from build123d import *

# Parameters (mm, degrees)
SKETCH1_R           = 48.26
BOSS_EXTRUDE1_DEPTH = 8.89
SKETCH3_R           = 1.7145
CUT_EXTRUDE1_DEPTH  = 3.81
SKETCH4_R           = 21.0185
CUT_EXTRUDE2_DEPTH  = 8.89
CUT_EXTRUDE3_DEPTH  = 99.56230669
BOSS_EXTRUDE2_START = -1.905
SKETCH8_R           = 2
BOSS_EXTRUDE2_DEPTH = 1.905
SKETCH9_R           = 23.622
CUT_EXTRUDE4_DEPTH  = 7.0104


with BuildPart() as part:
    # Sketch1 → Boss-Extrude1 (new body)
    with BuildSketch(Plane.XY):
        with Locations((21.15, -21.15)):
            Circle(SKETCH1_R)
    extrude(amount=BOSS_EXTRUDE1_DEPTH)

    # Sketch3 → Cut-Extrude1 (cut)
    with BuildSketch(Plane.XY.offset(8.89)):
        with Locations((25.240891907, 16.090983183)):
            Circle(SKETCH3_R)
        with Locations((34.034368653, 14.02981338)):
            Circle(SKETCH3_R)
        with Locations((42.079052724, 9.924120696)):
            Circle(SKETCH3_R)
        with Locations((48.907416326, 4.012513068)):
            Circle(SKETCH3_R)
        with Locations((54.122619785, -3.361448357)):
            Circle(SKETCH3_R)
        with Locations((57.421574432, -11.769215746)):
            Circle(SKETCH3_R)
        with Locations((58.612557015, -20.722160217)):
            Circle(SKETCH3_R)
        with Locations((57.626351956, -29.699969182)):
            Circle(SKETCH3_R)
        with Locations((54.520273906, -38.180885015)):
            Circle(SKETCH3_R)
        with Locations((49.474836834, -45.672027717)):
            Circle(SKETCH3_R)
        with Locations((42.783263201, -51.738039301)):
            Circle(SKETCH3_R)
        with Locations((34.834442945, -56.026385224)):
            Circle(SKETCH3_R)
        with Locations((26.090332605, -58.287842408)):
            Circle(SKETCH3_R)
        with Locations((17.059108093, -58.390983183)):
            Circle(SKETCH3_R)
        with Locations((8.265631347, -56.32981338)):
            Circle(SKETCH3_R)
        with Locations((0.220947276, -52.224120696)):
            Circle(SKETCH3_R)
        with Locations((-6.607416326, -46.312513068)):
            Circle(SKETCH3_R)
        with Locations((-11.822619785, -38.938551643)):
            Circle(SKETCH3_R)
        with Locations((-15.121574432, -30.530784254)):
            Circle(SKETCH3_R)
        with Locations((-16.312557015, -21.577839783)):
            Circle(SKETCH3_R)
        with Locations((-15.326351956, -12.600030818)):
            Circle(SKETCH3_R)
        with Locations((-12.220273906, -4.119114985)):
            Circle(SKETCH3_R)
        with Locations((-7.174836834, 3.372027717)):
            Circle(SKETCH3_R)
        with Locations((-0.483263201, 9.438039301)):
            Circle(SKETCH3_R)
        with Locations((7.465557055, 13.726385224)):
            Circle(SKETCH3_R)
        with Locations((16.209667395, 15.987842408)):
            Circle(SKETCH3_R)
    extrude(amount=-CUT_EXTRUDE1_DEPTH, mode=Mode.SUBTRACT)

    # Sketch4 → Cut-Extrude2 (cut)
    with BuildSketch(Plane.XY.offset(8.89)):
        with Locations((21.15, -21.15)):
            Circle(SKETCH4_R)
    extrude(amount=-CUT_EXTRUDE2_DEPTH, mode=Mode.SUBTRACT)

    # Sketch5 → Cut-Extrude3 (cut, through all)
    with BuildSketch(Plane(origin=(0, 0, 0), x_dir=(-1, 0, 0), z_dir=(0, 0, -1))):
        with BuildLine():
            ThreePointArc((-24.96, 23.3), (-21.15, 19.49), (-17.34, 23.3))
            Line((-17.34, 23.3), (-17.34, 26.959370189))
            ThreePointArc((-17.34, 26.959370189), (-21.15, 27.11), (-24.96, 26.959370189))
            Line((-24.96, 26.959370189), (-24.96, 23.3))
        make_face()
        with BuildLine():
            Line((-65.6, -17.34), (-69.259370189, -17.34))
            ThreePointArc((-69.259370189, -17.34), (-69.41, -21.15), (-69.259370189, -24.96))
            Line((-69.259370189, -24.96), (-65.6, -24.96))
            ThreePointArc((-65.6, -24.96), (-61.79, -21.15), (-65.6, -17.34))
        make_face()
        with BuildLine():
            Line((-24.96, -65.6), (-24.96, -69.259370189))
            ThreePointArc((-24.96, -69.259370189), (-21.15, -69.41), (-17.34, -69.259370189))
            Line((-17.34, -69.259370189), (-17.34, -65.6))
            ThreePointArc((-17.34, -65.6), (-21.15, -61.79), (-24.96, -65.6))
        make_face()
        with BuildLine():
            ThreePointArc((27.11, -21.15), (27.072327844, -19.243511779), (26.959370189, -17.34))
            Line((26.959370189, -17.34), (23.3, -17.34))
            ThreePointArc((23.3, -17.34), (19.49, -21.15), (23.3, -24.96))
            Line((23.3, -24.96), (26.959370189, -24.96))
            ThreePointArc((26.959370189, -24.96), (27.072327844, -23.056488221), (27.11, -21.15))
        make_face()
    extrude(amount=-CUT_EXTRUDE3_DEPTH, mode=Mode.SUBTRACT)

    # Sketch8 → Boss-Extrude2 (add)
    # profile 1 of 4: a face of its own
    with BuildSketch(Plane.XY.offset(8.89).offset(BOSS_EXTRUDE2_START)):
        with BuildLine():
            ThreePointArc((-26.959370189, -17.34), (-27.11, -21.15), (-26.959370189, -24.96))
            Line((-26.959370189, -24.96), (-23.3, -24.96))
            ThreePointArc((-23.3, -24.96), (-19.49, -21.15), (-23.3, -17.34))
            Line((-23.3, -17.34), (-26.959370189, -17.34))
        make_face()
        with Locations((-23.3, -21.15)):
            Circle(SKETCH8_R, mode=Mode.SUBTRACT)
    # profile 2 of 4: a face of its own
    with BuildSketch(Plane.XY.offset(8.89).offset(BOSS_EXTRUDE2_START)):
        with BuildLine():
            ThreePointArc((24.96, 26.959370189), (21.15, 27.11), (17.34, 26.959370189))
            Line((17.34, 26.959370189), (17.34, 23.3))
            ThreePointArc((17.34, 23.3), (21.15, 19.49), (24.96, 23.3))
            Line((24.96, 23.3), (24.96, 26.959370189))
        make_face()
        with Locations((21.15, 23.3)):
            Circle(SKETCH8_R, mode=Mode.SUBTRACT)
    # profile 3 of 4: a face of its own
    with BuildSketch(Plane.XY.offset(8.89).offset(BOSS_EXTRUDE2_START)):
        with BuildLine():
            ThreePointArc((69.259370189, -24.96), (69.41, -21.15), (69.259370189, -17.34))
            Line((69.259370189, -17.34), (65.6, -17.34))
            ThreePointArc((65.6, -17.34), (61.79, -21.15), (65.6, -24.96))
            Line((65.6, -24.96), (69.259370189, -24.96))
        make_face()
        with Locations((65.6, -21.15)):
            Circle(SKETCH8_R, mode=Mode.SUBTRACT)
    # profile 4 of 4: a face of its own
    with BuildSketch(Plane.XY.offset(8.89).offset(BOSS_EXTRUDE2_START)):
        with BuildLine():
            ThreePointArc((17.34, -69.259370189), (21.15, -69.41), (24.96, -69.259370189))
            Line((24.96, -69.259370189), (24.96, -65.6))
            ThreePointArc((24.96, -65.6), (21.15, -61.79), (17.34, -65.6))
            Line((17.34, -65.6), (17.34, -69.259370189))
        make_face()
        with Locations((21.15, -65.6)):
            Circle(SKETCH8_R, mode=Mode.SUBTRACT)
    extrude(amount=BOSS_EXTRUDE2_DEPTH)

    # Sketch9 → Cut-Extrude4 (cut)
    with BuildSketch(Plane(origin=(0, 0, 0), x_dir=(-1, 0, 0), z_dir=(0, 0, -1))):
        with Locations((-21.15, -21.15)):
            Circle(SKETCH9_R)
    extrude(amount=-CUT_EXTRUDE4_DEPTH, mode=Mode.SUBTRACT)


solid = part.part
Can you work these out from the model? Positions are in its coordinate system, mm. A direction names the side the tool comes from. Give positions to 0.01 mm unless a question says otherwise; leave off trailing zeros. Write each loop counter-clockwise with the first axis right and the second up, starting at its lowest first coordinate (ties: lowest second). Pieces come first, ordered by that corner, then holes. Notation, with made-up numbers: (38, 73) -> (79, 73) arc R12 ccw to (79, 87) -> close; hole circle Ø11 at (47, 65.5). An arc over 180 degrees is marked (long way). Answer as a JSON object with one key per item and string values. Group by question number.
Item 1: For faces 4 (the face through (-19.49, -21.07, 3.44)), 5 (the face through (54, -38, 5.08)), 6 (the face through (61.79, -21.23, 3.44)), 7 (the face through (17.34, -67, 3)), 8 (the face through (24.96, 25, 3)), which set-ups out of +Z, -Z, +X, -X, +Y, -Y let a thin tool reach every point of the face, with its end or its side?
Item 2: Suppose I cut it at A-A (x = 21.15). Please give me the cut outline in (y, z) (1 decimal).
Item 3: I'm going to push flat-ended pins straight in: P1, Ø3, axis at x = -11.82, y = -38.94, coming from the +Z side; P2, Ø4, axis at y = 10.5, z = 7, coming from the -X side; P3, Ø10, axis at x = 31.5, y = -6, coming from the -Z side. Where does each tip first touch, or does it pass through?
Item 4: Suppose I cut it at B-B (y = -34). Please give me the cut outline in (x, z), plus the area to 3 significant figures.
Item 5: Please list where these lines run through material, in increasing order: line 1 (Y direction, x = 42.5, z = 8.25); line 2 (X direction, y = -29, z = 5.25); line 3 (Y direction, x = 34, z = 5.5). Write a range as [from, to].
Item 6: We'd pull the mould along Y, two halves only. Please class faces 1 (the face through (40.366, 10, 7.012)), 2 (the face through (42, -31, 8.89)), 3 (the face through (60.196, -21.379, 7.012)): +Y half, -Y half, draft (parallel to the pull), parting line (faces both ways), or undercut.
Findings:
{
 "1": {"face 4": "-Z, -X", "face 5": "+Z", "face 6": "-Z, +X", "face 7": "-Z, -Y", "face 8": "-Z, +Y"},
 "2": {"outline": "(-69.4, 7) -> (-67.6, 7) -> (-67.6, 8.9) -> (-69.4, 8.9) -> close; (-63.6, 7) -> (-61.8, 7) -> (-61.8, 0) -> (-44.8, 0) -> (-44.8, 7) -> (-42.2, 7) -> (-42.2, 8.9) -> (-63.6, 8.9) -> close; (-0.1, 7) -> (2.5, 7) -> (2.5, 0) -> (19.5, 0) -> (19.5, 7) -> (21.3, 7) -> (21.3, 8.9) -> (-0.1, 8.9) -> close; (25.3, 7) -> (27.1, 7) -> (27.1, 8.9) -> (25.3, 8.9) -> close"},
 "3": {"P1": "stops at z = 5.08", "P2": "stops at x = -16.93", "P3": "stops at z = 7.01"},
 "4": {"outline": "(-25.37, 0) -> (1.33, 0) -> (1.33, 7.01) -> (4.52, 7.01) -> (4.52, 8.89) -> (-25.37, 8.89) -> close; (37.78, 7.01) -> (40.97, 7.01) -> (40.97, 0) -> (67.67, 0) -> (67.67, 8.89) -> (37.78, 8.89) -> close", "area": "487 mm²"},
 "5": {"line 1": "y = [-64.43, -53.43], [-50.05, 8.26], [11.59, 22.13]", "line 2": "x = [-26.47, -15.89], [-14.35, -1.13], [43.43, 56.06], [59.19, 68.77]", "line 3": "y = [-67.67, -57.52], [-54.53, -40.97], [-1.33, 12.32], [15.74, 25.37]"},
 "6": {"face 1": "undercut", "face 2": "draft", "face 3": "undercut"}
}
